CAD build for the part. Positions are in the model's coordinates, mm. Give positions to 0.01 mm unless a question says otherwise; leave off trailing zeros. Loops run counter-clockwise (first coordinate to the right, second up) from the corner with the lowest first, then second, coordinate; pieces in that order, holes last.
Item 1: Saw through at C-C on y = 5. Give the cut face in (x, z).
Item 2: Saw through at A-A on z = 2.25. Give the cut face in (x, y).
Item 3: Probe probe 1 along Y at (x, z) = (-30, 1.4); probe 2 along X at (y, z) = (6.5, 0.45); probe 3 along X at (y, z) = (-7, 1.3). List the from-to ranges inside material, lowest first.
Item 4: Saw through at D-D on y = -9.5. Give the cut face in (x, z), plus the area to 3 significant figures.
Item 5: Saw through at B-B on x = -30. Give the cut face in (y, z).
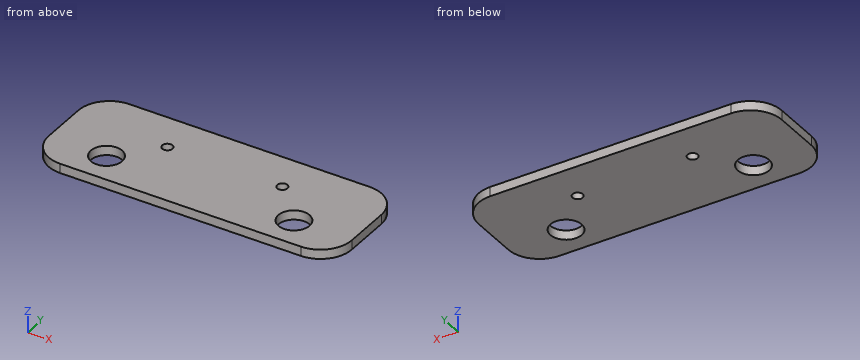
from build123d import *

# Parameters (mm, degrees)
SKETCH_1_W          = 91
SKETCH_1_H          = 35
EXTRUDE_2_DEPTH     = 3
SKETCH_2_R          = 1.25
CUT_EXTRUDE_1_DEPTH = 3
SKETCH_3_W          = 91
SKETCH_3_H          = 3
EXTRUDE_3_DEPTH     = 12
EXTRUDE_4_DEPTH     = 3
SKETCH_6_R          = 1.25
CUT_EXTRUDE_2_DEPTH = 3
SKETCH_7_W          = 27
SKETCH_7_H          = 35
EXTRUDE_5_DEPTH     = 3
SKETCH_8_R          = 1.25
CUT_EXTRUDE_3_DEPTH = 3
CUT_EXTRUDE_4_DEPTH = 57.669628421
SKETCH_10_R         = 5
CUT_EXTRUDE_5_DEPTH = 57.669628421
FILLET_1_R          = 10
SKETCH_11_R         = 1.65
CUT_EXTRUDE_6_DEPTH = 10
EXTRUDE_START       = -3
SKETCH_12_R         = 1.25
EXTRUDE_6_DEPTH     = 3


with BuildPart() as part:
    # 草图1 → 凸台-拉伸2 (new body)
    with BuildSketch(Plane.XY):
        Rectangle(SKETCH_1_W, SKETCH_1_H)
    extrude(amount=EXTRUDE_2_DEPTH)

    # 草图2 → 切除-拉伸1 (cut)
    with BuildSketch(Plane(origin=(0, 0, 0), x_dir=(-1, 0, 0), z_dir=(0, 0, -1))):
        with Locations((-22.5, 5)):
            Circle(SKETCH_2_R)
        with Locations(Location((22.5, 5, 0), (0, 0, 180))):
            Circle(SKETCH_2_R)
    extrude(amount=-CUT_EXTRUDE_1_DEPTH, mode=Mode.SUBTRACT)

    # 草图3 → 凸台-拉伸3 (add)
    with BuildSketch(Plane(origin=(0, 0, 0), x_dir=(-1, 0, 0), z_dir=(0, 0, -1))):
        with Locations((0, 16)):
            Rectangle(SKETCH_3_W, SKETCH_3_H)
    extrude(amount=EXTRUDE_3_DEPTH)

    # 草图4 → 凸台-拉伸4 (add)
    with BuildSketch(Plane(origin=(45.5, 0, 0), x_dir=(0, 0, -1), z_dir=(1, 0, 0))):
        Polygon((12, 17.5), (24, 17.5), (24, -17.5), (-3, -17.5), (-3, 17.5), align=None)
    extrude(amount=EXTRUDE_4_DEPTH)

    # 草图6 → 切除-拉伸2 (cut)
    with BuildSketch(Plane.ZY.offset(-45.5)):
        with Locations((-20, 9.5)):
            Circle(SKETCH_6_R)
        with Locations(Location((-20, -15.5, 0), (0, 0, 180))):
            Circle(SKETCH_6_R)
    extrude(amount=-CUT_EXTRUDE_2_DEPTH, mode=Mode.SUBTRACT)

    # 草图7 → 凸台-拉伸5 (add)
    with BuildSketch(Plane.ZY.offset(45.5)):
        with Locations((-10.5, 0)):
            Rectangle(SKETCH_7_W, SKETCH_7_H)
    extrude(amount=EXTRUDE_5_DEPTH)

    # 草图8 → 切除-拉伸3 (cut)
    with BuildSketch(Plane.ZY.offset(48.5)):
        with Locations((-20, 9.5)):
            Circle(SKETCH_8_R)
        with Locations(Location((-20, -15.5, 0), (0, 0, 180))):
            Circle(SKETCH_8_R)
    extrude(amount=-CUT_EXTRUDE_3_DEPTH, mode=Mode.SUBTRACT)

    # 草图9 → 切除-拉伸4 (cut)
    with BuildSketch(Plane(origin=(0, 0, 0), x_dir=(-1, 0, 0), z_dir=(0, 0, -1))):
        Polygon((-104.540404499, 43.487772061), (97.135742415, 67.997211031), (114.089056769, -71.503294087), (-87.587090144, -96.012733056), align=None)
    extrude(amount=CUT_EXTRUDE_4_DEPTH, mode=Mode.SUBTRACT)

    # 草图10 → 切除-拉伸5 (cut)
    with BuildSketch(Plane.XY.offset(3)):
        with Locations((-30, -7.5)):
            Circle(SKETCH_10_R)
        with Locations(Location((30, -7.5, 0), (0, 0, 180))):
            Circle(SKETCH_10_R)
    extrude(amount=-CUT_EXTRUDE_5_DEPTH, mode=Mode.SUBTRACT)

    # 圆角1
    fillet_1_edges = [part.edges().sort_by_distance(p)[0] for p in [
        (48.5, -17.5, 1.5),
        (-48.5, 17.5, 1.5),
        (-48.5, -17.5, 1.5),
        (48.5, 17.5, 1.5),
    ]]
    fillet(fillet_1_edges, radius=FILLET_1_R)

    # 草图11 → 切除-拉伸6 (cut)
    with BuildSketch(Plane.XY.offset(3)):
        with Locations((18.4, 5)):
            Circle(SKETCH_11_R)
        with Locations(Location((-18.4, 5, 0), (0, 0, 180))):
            Circle(SKETCH_11_R)
    extrude(amount=-CUT_EXTRUDE_6_DEPTH, mode=Mode.SUBTRACT)

    # 草图12 → 凸台-拉伸6 (add)
    with BuildSketch(Plane.XY.offset(3).offset(EXTRUDE_START)):
        with Locations((22.5, 5)):
            Circle(SKETCH_12_R)
        with Locations((-22.5, 5)):
            Circle(SKETCH_12_R)
    extrude(amount=EXTRUDE_6_DEPTH)


solid = part.part
Results below:
1. outline: (-48.5, 0) - (-20.05, 0) - (-20.05, 3) - (-48.5, 3) - close; (-16.75, 0) - (16.75, 0) - (16.75, 3) - (-16.75, 3) - close; (20.05, 0) - (48.5, 0) - (48.5, 3) - (20.05, 3) - close
2. outline: (-48.5, -7.5) arc R10 ccw to (-38.5, -17.5) - (38.5, -17.5) arc R10 ccw to (48.5, -7.5) - (48.5, 7.5) arc R10 ccw to (38.5, 17.5) - (-38.5, 17.5) arc R10 ccw to (-48.5, 7.5) - close; hole circle Ø10 at (-30, -7.5); hole circle Ø3.3 at (-18.4, 5); hole circle Ø3.3 at (18.4, 5); hole circle Ø10 at (30, -7.5)
3. probe 1: y = -17.5 to -12.5, -2.5 to 17.5
3. probe 2: x = -48.5 to -19.09, -17.71 to 17.71, 19.09 to 48.5
3. probe 3: x = -48.5 to -34.97, -25.03 to 25.03, 34.97 to 48.5
4. outline: (-48.3, 0) - (-34.58, 0) - (-34.58, 3) - (-48.3, 3) - close; (-25.42, 0) - (25.42, 0) - (25.42, 3) - (-25.42, 3) - close; (34.58, 0) - (48.3, 0) - (48.3, 3) - (34.58, 3) - close
4. area: 235 mm2
5. outline: (-17.5, 0) - (-12.5, 0) - (-12.5, 3) - (-17.5, 3) - close; (-2.5, 0) - (17.5, 0) - (17.5, 3) - (-2.5, 3) - close
